```python
from build123d import *

# Parameters (mm, degrees)
SKETCH1_W           = 8.7
SKETCH1_H           = 6
SKETCH1_H_2         = 4.5
SKETCH1_W_2         = 3.5
SKETCH1_R           = 1
BOSS_EXTRUDE1_DEPTH = 2
FILLET1_R           = 0.5
SKETCH2_W           = 8
SKETCH2_H           = 4.5
SKETCH2_W_2         = 5
SKETCH2_H_2         = 4
BOSS_EXTRUDE2_DEPTH = 3
SKETCH3_W           = 5
SKETCH3_H           = 4.4
BOSS_EXTRUDE3_DEPTH = 1.2


with BuildPart() as part:
    # Sketch1 → Boss-Extrude1 (new body)
    # profile 1 of 5: a face of its own
    with BuildSketch(Plane(origin=(0, 0, 0), x_dir=(1, 0, 0), z_dir=(0, 1, 0))):
        with Locations((0, 5.25)):
            Rectangle(SKETCH1_W, SKETCH1_H)
    # profile 2 of 5: a face of its own
    with BuildSketch(Plane(origin=(0, 0, 0), x_dir=(1, 0, 0), z_dir=(0, 1, 0))):
        Rectangle(SKETCH1_W, SKETCH1_H_2)
    # profile 3 of 5: a face of its own
    with BuildSketch(Plane(origin=(0, 0, 0), x_dir=(1, 0, 0), z_dir=(0, 1, 0))):
        with Locations((-6.1, 0)):
            Rectangle(SKETCH1_W_2, SKETCH1_H_2)
        with Locations(Location((-6, 0, 0), (0, 0, 270))):
            Circle(SKETCH1_R, mode=Mode.SUBTRACT)
    # profile 4 of 5: a face of its own
    with BuildSketch(Plane(origin=(0, 0, 0), x_dir=(1, 0, 0), z_dir=(0, 1, 0))):
        with Locations((6.1, 0)):
            Rectangle(SKETCH1_W_2, SKETCH1_H_2)
        with Locations(Location((6, 0, 0), (0, 0, 270))):
            Circle(SKETCH1_R, mode=Mode.SUBTRACT)
    # profile 5 of 5: a face of its own
    with BuildSketch(Plane(origin=(0, 0, 0), x_dir=(1, 0, 0), z_dir=(0, 1, 0))):
        with Locations((0, -5.25)):
            Rectangle(SKETCH1_W, SKETCH1_H)
    extrude(amount=BOSS_EXTRUDE1_DEPTH)

    # Fillet1
    fillet1_edges = [part.edges().sort_by_distance(p)[0] for p in [
        (-4.35, 1, -8.25),
        (4.35, 1, -8.25),
        (4.35, 1, -2.25),
        (7.85, 1, -2.25),
        (7.85, 1, 2.25),
        (4.35, 1, 2.25),
        (4.35, 1, 8.25),
        (-4.35, 1, 8.25),
        (-4.35, 1, 2.25),
        (-7.85, 1, 2.25),
        (-7.85, 1, -2.25),
        (-4.35, 1, -2.25),
    ]]
    fillet(fillet1_edges, radius=FILLET1_R)

    # Sketch2 → Boss-Extrude2 (add)
    with BuildSketch(Plane.XZ):
        with Locations((0, -5)):
            Rectangle(SKETCH2_W, SKETCH2_H)
        with Locations((0, 5.25)):
            Rectangle(SKETCH2_W_2, SKETCH2_H_2)
    extrude(amount=BOSS_EXTRUDE2_DEPTH)

    # Sketch3 → Boss-Extrude3 (add)
    with BuildSketch(Plane(origin=(0, 2, 0), x_dir=(1, 0, 0), z_dir=(0, 1, 0))):
        Rectangle(SKETCH3_W, SKETCH3_H)
    extrude(amount=BOSS_EXTRUDE3_DEPTH)


solid = part.part
```
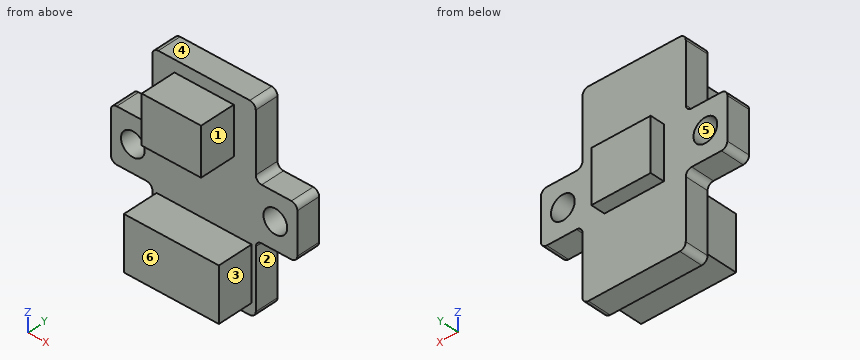
The listing builds one solid part. Answer for the finished solid, in the listing's coordinates (mm). Face numbers are marked on the shaded views. A direction names the side the tool comes from. Coordinates: 2 decimals unless noted, no trailing zeros. Loops run counter-clockwise (first coordinate to the right, second up) from the corner with the lowest first, then second, coordinate; pieces in that order, holes last. Notation, with made-up numbers: M 51.5,-36 L 89.5,-36 A7 cw 89.5,-24 Z; hole C 54.5,-38.75 d7. An arc over 180 degrees is marked long. Answer as CSV lines item,"result". Start each with the question number.
(1) The part is cut by section D-D (z = 0). Give the vertices of the cut face in (x, y), and give its area (3 significant figures).
(2) The part is cut by section A-A (y = -2.5). Give the vertices of the cut face in (x, z).
(3) The part is cut by section C-C (y = 0.75). Give the vertices of the cut face in (x, z).
(4) For the marked faces 1, 2 and 3, determine the directions among +Z, -Z, +X, -X, +Y, -Y from which every point of the face is accessible in a straight line to the end or side of a thin tool.
(5) The mould has two halves that part along Z. Classify the marked faces 4, 5 and 6: pulls with the +Z half, pulls with the -Z half, needs draft (parallel to the pull), parting line crosses it, or undercut.
(6) Given pin 1 (1 mm diameter, centred on x = 6.5, y = 1.5, fed in from -Z); pin 2 (1.5 mm diameter, centred on x = 1, y = -1.5, fed in from -Z); pin 3 (2 mm diameter, centred on y = 1.5, z = -5.5, fed in from -X); pin 4 (5 mm diameter, centred on x = -3.5, z = -1.5, fed in from -Y), each flat-ended and moving along its own axis, determine where each tip first touches the part or whether it passes through.
(7) Find the intervals of material crossed by L1, parallel to X at y = 1.1, z = 0; L2, parallel to X at y = 1.25, z = 6.25; L3, parallel to Y at x = -1.75, z = -5.25, in increasing order. Write a range as [from, to].
(8) The part is cut by section B-B (x = -6). Give the vertices of the cut face in (y, z), and give its area (3 significant figures).
Determined:
1,outline,"M -7.85,0 L -7,0 L -7,2 L -7.85,2 Z; M -5,0 L 5,0 L 5,2 L 2.5,2 L 2.5,3.2 L -2.5,3.2 L -2.5,2 L -5,2 Z; M 7,0 L 7.85,0 L 7.85,2 L 7,2 Z"
1,area,"29.4 mm2"
2,outline,"M -4,-7.25 L 4,-7.25 L 4,-2.75 L -4,-2.75 Z; M -2.5,3.25 L 2.5,3.25 L 2.5,7.25 L -2.5,7.25 Z"
3,outline,"M -7.85,-1.75 A0.5 ccw -7.35,-2.25 L -4.85,-2.25 A0.5 cw -4.35,-2.75 L -4.35,-7.75 A0.5 ccw -3.85,-8.25 L 3.85,-8.25 A0.5 ccw 4.35,-7.75 L 4.35,-2.75 A0.5 cw 4.85,-2.25 L 7.35,-2.25 A0.5 ccw 7.85,-1.75 L 7.85,1.75 A0.5 ccw 7.35,2.25 L 4.85,2.25 A0.5 cw 4.35,2.75 L 4.35,7.75 A0.5 ccw 3.85,8.25 L -3.85,8.25 A0.5 ccw -4.35,7.75 L -4.35,2.75 A0.5 cw -4.85,2.25 L -7.35,2.25 A0.5 ccw -7.85,1.75 Z; hole C -6,0 d2; hole C 6,0 d2"
4,face 1,"+Z, +X, -Y"
4,face 2,"-Z, +X, +Y, -Y"
4,face 3,"+Z, -Z, +X, -Y"
5,face 4,"pulls with the +Z half"
5,face 5,"undercut"
5,face 6,"needs draft"
6,pin 1,"z = -2.25"
6,pin 2,"z = -7.25"
6,pin 3,"x = -4.35"
6,pin 4,"y = -3"
7,L1,"[-7.85, -7], [-5, 5], [7, 7.85]"
7,L2,"[-4.35, 4.35]"
7,L3,"[-3, 2]"
8,outline,"M 0,-2.25 L 2,-2.25 L 2,-1 L 0,-1 Z; M 0,1 L 2,1 L 2,2.25 L 0,2.25 Z"
8,area,"5.00 mm2"
